```python
from build123d import *

# Parameters (mm, degrees)
SKETCH1_W           = 40
SKETCH1_H           = 20
BOSS_EXTRUDE1_DEPTH = 2
SKETCH2_W           = 40
SKETCH2_H           = 2
BOSS_EXTRUDE2_DEPTH = 20
SKETCH4_R           = 5
SKETCH4_R_2         = 1
CUT_EXTRUDE2_DEPTH  = 36.832945734
SKETCH5_R           = 2
CUT_EXTRUDE3_DEPTH  = 32.368774283
SKETCH6_W           = 4.431073847
SKETCH6_H           = 18
BOSS_EXTRUDE3_DEPTH = 20
CHAMFER1_SIZE       = 15
SKETCH7_W           = 13
SKETCH7_H           = 2.5
BOSS_EXTRUDE4_DEPTH = 15
FILLET1_R           = 6
SKETCH8_R           = 2
CUT_EXTRUDE4_DEPTH  = 40.37003937
MIRROR1_START       = 4.5
MIRROR1_OUTLINE_R   = 2
MIRROR1_DEPTH       = 2.5
MIRROR1_START_2     = 2
MIRROR1_2_OUTLINE_W = 4.431073847
MIRROR1_2_OUTLINE_H = 18
MIRROR1_2_DEPTH     = 2.5
MIRROR1_START_3     = 15.568926153
MIRROR1_3_DEPTH     = 4.431073847


with BuildPart() as part:
    # Sketch1 → Boss-Extrude1 (new body)
    with BuildSketch(Plane(origin=(0, 0, 0), x_dir=(1, 0, 0), z_dir=(0, 1, 0))):
        Rectangle(SKETCH1_W, SKETCH1_H)
    extrude(amount=BOSS_EXTRUDE1_DEPTH)

    # Sketch2 → Boss-Extrude2 (add)
    with BuildSketch(Plane(origin=(0, 2, 0), x_dir=(1, 0, 0), z_dir=(0, 1, 0))):
        with Locations((0, 9)):
            Rectangle(SKETCH2_W, SKETCH2_H)
    extrude(amount=BOSS_EXTRUDE2_DEPTH)

    # Sketch4 → Cut-Extrude2 (cut, through all)
    with BuildSketch(Plane(origin=(0, 0, -10), x_dir=(-1, 0, 0), z_dir=(0, 0, -1))):
        with Locations((0, 13.5)):
            Circle(SKETCH4_R)
        with Locations((-9.5, 16.5)):
            Circle(SKETCH4_R_2)
        with Locations((9.5, 16.5)):
            Circle(SKETCH4_R_2)
    extrude(amount=-CUT_EXTRUDE2_DEPTH, mode=Mode.SUBTRACT)

    # Sketch5 → Cut-Extrude3 (cut, through all)
    with BuildSketch(Plane.XZ):
        with Locations(Location((0, 0, 0), (0, 0, 270))):
            Circle(SKETCH5_R)
    extrude(amount=-CUT_EXTRUDE3_DEPTH, mode=Mode.SUBTRACT)

    # Sketch6 → Boss-Extrude3 (add)
    with BuildSketch(Plane(origin=(0, 2, 0), x_dir=(1, 0, 0), z_dir=(0, 1, 0))):
        with Locations((-17.784463076, -1)):
            Rectangle(SKETCH6_W, SKETCH6_H)
    extrude(amount=BOSS_EXTRUDE3_DEPTH)

    # Chamfer1
    chamfer1_edges = [part.edges().sort_by_distance(p)[0] for p in [
        (-17.784463077, 22, 10),
    ]]
    chamfer(chamfer1_edges, length=CHAMFER1_SIZE)

    # Sketch7 → Boss-Extrude4 (add)
    with BuildSketch(Plane.ZY.offset(20)):
        with Locations((0, 5.75)):
            Rectangle(SKETCH7_W, SKETCH7_H)
    extrude(amount=BOSS_EXTRUDE4_DEPTH)

    # Fillet1
    # the kernel refuses this fillet: 6 mm, written as the material it adds along each edge
    with BuildSketch(Plane(origin=(-20, 4.5, 6.5), x_dir=(0, 0, 1), z_dir=(0, 1, 0)), Plane(origin=(-20, 7, -6.5), x_dir=(0, 0, -1), z_dir=(0, -1, 0))) as fillet1_piece_1:
        with BuildLine():
            CenterArc((6, -5.454356057), FILLET1_R, 114.624318352, 65.375681648)
            Line((0, -5.454356057), (0, 0))
            Line((0, 0), (3.5, 0))
        make_face()
    extrude(amount=2.5)
    # the kernel refuses this fillet: 6 mm, written as the material it takes off along each edge
    with BuildSketch(Plane(origin=(-35, -10.5, 6.5), x_dir=(1, 0, 0), z_dir=(0, 1, 0))) as fillet1_2_piece_1:
        with BuildLine():
            CenterArc((FILLET1_R, FILLET1_R), FILLET1_R, 180, 90)
            Line((0, FILLET1_R), (0, 0))
            Line((0, 0), (FILLET1_R, 0))
        make_face()
    extrude(amount=32.5, mode=Mode.SUBTRACT)
    with BuildSketch(Plane(origin=(-35, 22, -6.5), x_dir=(0, 0, 1), z_dir=(0, -1, 0))) as fillet1_2_piece_2:
        with BuildLine():
            CenterArc((FILLET1_R, -FILLET1_R), FILLET1_R, 90, 90)
            Line((0, -FILLET1_R), (0, 0))
            Line((0, 0), (FILLET1_R, 0))
        make_face()
    extrude(amount=32.5, mode=Mode.SUBTRACT)

    # Sketch8 → Cut-Extrude4 (cut, through all)
    with BuildSketch(Plane(origin=(0, 7, 0), x_dir=(1, 0, 0), z_dir=(0, 1, 0))):
        with Locations(Location((-29, 0, 0), (0, 0, 270))):
            Circle(SKETCH8_R)
    extrude(amount=-CUT_EXTRUDE4_DEPTH, mode=Mode.SUBTRACT)

    # Mirror1: read off the stored shape, not the designer's step
    # Mirror1 outline → Mirror1 (add)
    with BuildSketch(Plane(origin=(0, 0, 0), x_dir=(1, 0, 0), z_dir=(0, 1, 0)).offset(MIRROR1_START)):
        with BuildLine():
            Line((20, 6.5), (20, 8))
            Line((20, 8), (15.568926153, 8))
            Line((15.568926153, 8), (15.568926153, -10))
            Line((15.568926153, -10), (20, -10))
            Line((20, -10), (20, -6.5))
            Line((20, -6.5), (29, -6.5))
            ThreePointArc((29, -6.5), (33.242640687, -4.742640687), (35, -0.5))
            Line((35, -0.5), (35, 0.5))
            ThreePointArc((35, 0.5), (33.242640687, 4.742640687), (29, 6.5))
            Line((29, 6.5), (20, 6.5))
        make_face()
        with Locations((29, 0)):
            Circle(MIRROR1_OUTLINE_R, mode=Mode.SUBTRACT)
    extrude(amount=MIRROR1_DEPTH)

    # Mirror1 2 outline → Mirror1 2 (add)
    with BuildSketch(Plane(origin=(0, 0, 0), x_dir=(1, 0, 0), z_dir=(0, 1, 0)).offset(MIRROR1_START_2)):
        with Locations((17.784463076, -1)):
            Rectangle(MIRROR1_2_OUTLINE_W, MIRROR1_2_OUTLINE_H)
    extrude(amount=MIRROR1_2_DEPTH)

    # Mirror1 3 outline → Mirror1 3 (add)
    with BuildSketch(Plane.YZ.offset(MIRROR1_START_3)):
        Polygon((7, -8), (22, -8), (22, -5), (7, 10), align=None)
    extrude(amount=MIRROR1_3_DEPTH)


solid = part.part
```
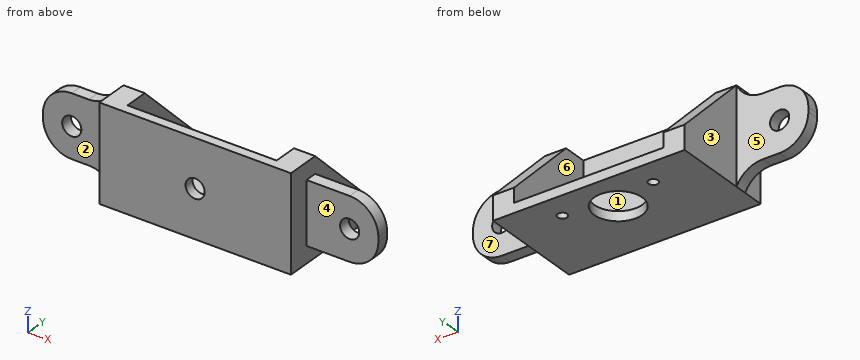
Here's how the part is built. I have some questions about the finished solid (model axes, mm). Face numbers are marked on the shaded views. A direction names the side the tool comes from. Give positions to 0.01 mm unless a question says otherwise; leave off trailing zeros. Order: outer loops, then holes, each group sorted by start corner. A loop starts at its lowest first (then second) coordinate and runs counter-clockwise, first axis right, second up. Notation, with made-up numbers: (-8, 41.5) -> (19, 41.5) arc R22 ccw to (19, 65.5) -> close; hole circle Ø2 at (84, -33). An arc over 180 degrees is marked (long way). Use CSV: the item, a comma, the result in double quotes. Start each with the question number.
Item 1: On a 3-axis mill with a long thin cutter (end or side, diameter ignored), from which of +Z, -Z, +X, -X, +Y, -Y can I reach the whole of each face in a straight line? I mean the marked faces 4, 5, 6 and 7. Say none if no direction works.
Item 2: I'm going to push flat-ended pins straight in: P1, Ø9, axis at y = 17, z = -0.5, coming from the +X side; P2, Ø6, axis at x = 2, y = 11.5, coming from the +Z side; P3, Ø5, axis at x = 29, z = 0, coming from the -Y side. Where does each tip first touch, or does it pass through?
Item 3: Suppose I cut it at C-C (y = 16.5). List the corners of the cut face in (x, z) for me.
Item 4: Thinking about a two-plate mould opening in X: for the marked faces 1, 2 and 3, which applies, pulls with the +X half, pulls with the -X half, needs draft (parallel to the pull), parting line crosses it, or undercut?
Item 5: Suppose I cut it at A-A (y = 13.5). List the corners of the cut face in (x, z) for me.
Item 6: If I drill on probe 1 along X at (y, z) = (1.5, 0); probe 2 along Y at (x, z) = (9.5, -9.1); probe 3 along X at (y, z) = (7.5, 5.5), over which ranges is the centre line in solid material (lowest first)? Write a range as [from, to].
Item 7: Suppose I cut it at D-D (y = 5.5). List the corners of the cut face in (x, z) for me, and give its area (3 significant figures).
Item 8: Suppose I cut it at B-B (x = -3). List the corners of the cut face in (y, z) for me, and give its area (3 significant figures).
Answer block:
1,face 4,"+Z, -Z, +X, -Y"
1,face 5,"+Z, -Z, -X, +Y"
1,face 6,"+Z, +Y"
1,face 7,"+Z, -Z, +X, +Y"
2,P1,"stops at x = 20"
2,P2,"stops at z = -8"
2,P3,"stops at y = 4.5"
3,outline,"(-20, -10) -> (-10.5, -10) -> (-10.5, -8) -> (-15.57, -8) -> (-15.57, 0.5) -> (-20, 0.5) -> close; (-8.5, -10) -> (-4, -10) -> (-4, -8) -> (-8.5, -8) -> close; (4, -10) -> (8.5, -10) -> (8.5, -8) -> (4, -8) -> close; (10.5, -10) -> (20, -10) -> (20, 0.5) -> (15.57, 0.5) -> (15.57, -8) -> (10.5, -8) -> close"
4,face 1,"undercut"
4,face 2,"needs draft"
4,face 3,"pulls with the -X half"
5,outline,"(-20, -10) -> (-5, -10) -> (-5, -8) -> (-15.57, -8) -> (-15.57, 3.5) -> (-20, 3.5) -> close; (5, -10) -> (20, -10) -> (20, 3.5) -> (15.57, 3.5) -> (15.57, -8) -> (5, -8) -> close"
6,probe 1,"x = [-20, -2], [2, 20]"
6,probe 2,"y = [0, 15.5], [17.5, 22]"
6,probe 3,"x = [-20, -15.57], [15.57, 20]"
7,outline,"(-35, -0.5) arc R6 ccw to (-29, -6.5) -> (-25.45, -6.5) arc R6 cw to (-20, -10) -> (20, -10) -> (20, -6.5) -> (29, -6.5) arc R6 ccw to (35, -0.5) -> (35, 0.5) arc R6 ccw to (29, 6.5) -> (20, 6.5) -> (20, 10) -> (15.57, 10) -> (15.57, -8) -> (-15.57, -8) -> (-15.57, 10) -> (-20, 10) arc R6 cw to (-25.45, 6.5) -> (-29, 6.5) arc R6 ccw to (-35, 0.5) -> close; hole circle Ø4 at (-29, 0); hole circle Ø4 at (29, 0)"
7,area,"584 mm^2"
8,outline,"(0, -10) -> (9.5, -10) -> (9.5, -8) -> (2, -8) -> (2, 10) -> (0, 10) -> close; (17.5, -10) -> (22, -10) -> (22, -8) -> (17.5, -8) -> close"
8,area,"64.0 mm^2"
